Read the model definition and answer for the solid it produces. Units are mm, in the model's axes. Face numbers are marked on the shaded views. A direction names the side the tool comes from. Give positions to 0.01 mm unless a question says otherwise; leave off trailing zeros. Order: outer loops, then holes, each group sorted by start corner. A loop starts at its lowest first (then second) coordinate and runs counter-clockwise, first axis right, second up.
Item 1: Which of the six approach directions +Z, -Z, +X, -X, +Y, -Y give full straight-line access (tool end or side, diameter ignored) to the marked faces 1 and 2?
Item 2: A cutting plane is placed at C-C (y = 254). Write down the section's boundary in (x, z), plus the area to 3 significant figures.
Item 3: A cutting plane is placed at D-D (x = 83). Write down the section's boundary in (y, z), plus the area to 3 significant figures.
Item 4: Find the intervals of material crossed by line 1 along Y through (x, z) = (-2.5, 220.5); line 2 along Z through (x, y) = (109.5, 456.5); line 3 along X through (y, z) = (370.5, 295), in increasing order.
Item 5: Given pin 1 Ø6 at (x, z) = (-69, 212.5) entering from +Y; pin 2 Ø24 at (x, y) = (-17, 385.5) entering from -Z; pin 3 Ø2 at (x, y) = (81.5, 90.5) entering from -Z, each flat-ended and moving along its own axis, determine where each tip first touches the part or whether it passes through.
Item 6: A cutting plane is placed at B-B (z = 213). Write down the section's boundary in (x, y), plus the area to 3 significant figures.
Item 7: A cutting plane is placed at A-A (x = 6). Write down the section's boundary in (y, z), plus the area to 3 significant figures.
from build123d import *

# Parameters (mm, degrees)
SK_DOCKBASE_W         = 300
SK_DOCKBASE_H         = 129.6
EX_DOCKBASE_DEPTH     = 5
SK_DOCKWALL_W         = 300
SK_DOCKWALL_H         = 10
EX_DOCKWALL_DEPTH     = 500
SK_APRILTAG_W         = 80
SK_APRILTAG_H         = 80
EX_APRILTAG_DEPTH     = 1
SK_DOCKCONTACTS_W     = 26
SK_DOCKCONTACTS_H     = 20
EX_DOCKCONTACTS_DEPTH = 25


with BuildPart() as part:
    # SK_DockBase → EX_DockBase (new body)
    with BuildSketch(Plane(origin=(0, 0, 0), x_dir=(1, 0, 0), z_dir=(0, 1, 0))):
        with Locations((0, -240.8)):
            Rectangle(SK_DOCKBASE_W, SK_DOCKBASE_H)
    extrude(amount=EX_DOCKBASE_DEPTH)

    # SK_DockWall → EX_DockWall (add)
    with BuildSketch(Plane(origin=(0, 0, 0), x_dir=(1, 0, 0), z_dir=(0, 1, 0))):
        with Locations((0, -300.6)):
            Rectangle(SK_DOCKWALL_W, SK_DOCKWALL_H)
    extrude(amount=EX_DOCKWALL_DEPTH)

    # SK_AprilTag → EX_AprilTag (add)
    with BuildSketch(Plane.XY.offset(295.6)):
        with Locations((0, 400)):
            Rectangle(SK_APRILTAG_W, SK_APRILTAG_H)
    extrude(amount=-EX_APRILTAG_DEPTH)

    # SK_DockContacts → EX_DockContacts (add)
    with BuildSketch(Plane(origin=(0, 5, 0), x_dir=(1, 0, 0), z_dir=(0, 1, 0))):
        with Locations((64, -216)):
            Rectangle(SK_DOCKCONTACTS_W, SK_DOCKCONTACTS_H)
        with Locations((-64, -216)):
            Rectangle(SK_DOCKCONTACTS_W, SK_DOCKCONTACTS_H)
    extrude(amount=EX_DOCKCONTACTS_DEPTH)


solid = part.part
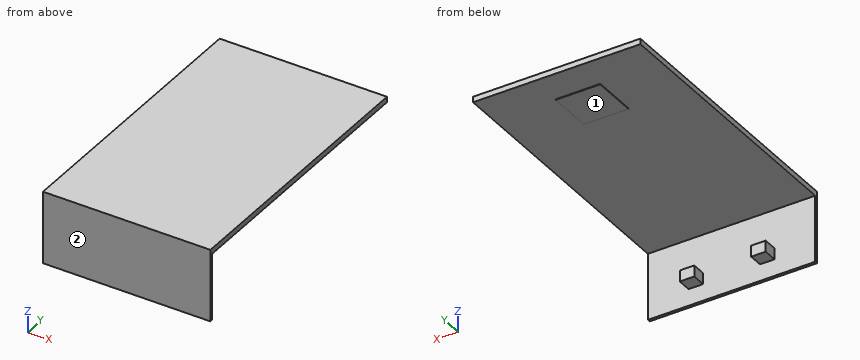
Response values:
1. face 1: -Z, +X, -X, +Y
1. face 2: +Z, -Z, +X, -X, -Y
2. outline: (-150, 295.6) - (150, 295.6) - (150, 305.6) - (-150, 305.6) - close
2. area: 3,000 mm2
3. outline: (0, 176) - (5, 176) - (5, 295.6) - (500, 295.6) - (500, 305.6) - (0, 305.6) - close
3. area: 5,600 mm2
4. line 1: y = 0 to 5
4. line 2: z = 295.6 to 305.6
4. line 3: x = -40 to 40
5. pin 1: stops at y = 30
5. pin 2: stops at z = 294.6
5. pin 3: stops at z = 295.6
6. outline: (-150, 0) - (150, 0) - (150, 5) - (77, 5) - (77, 30) - (51, 30) - (51, 5) - (-51, 5) - (-51, 30) - (-77, 30) - (-77, 5) - (-150, 5) - close
6. area: 2,800 mm2
7. outline: (0, 176) - (5, 176) - (5, 295.6) - (360, 295.6) - (360, 294.6) - (440, 294.6) - (440, 295.6) - (500, 295.6) - (500, 305.6) - (0, 305.6) - close
7. area: 5,680 mm2
